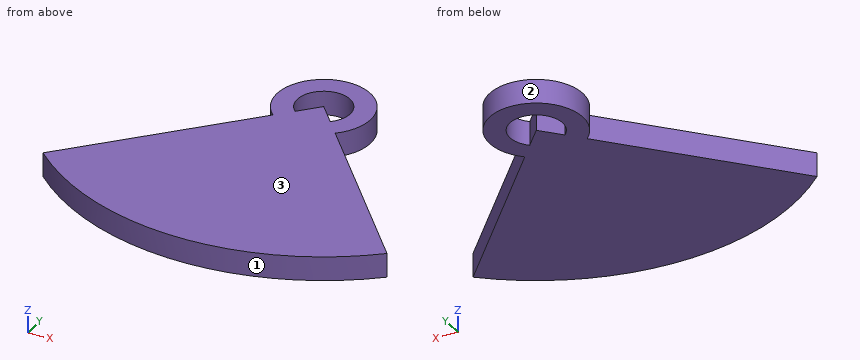
```python
from build123d import *

# Parameters (mm, degrees)
F1_DEPTH = 3
F6_DEPTH = 3


# Not quite as in the source:
# - the program builds the solid bodies; features that only make, move or delete a surface that nothing else refers to are left out


with BuildPart() as f1:
    # F0 (on Top) → F1 (new body)
    with BuildSketch(Plane.XY):
        with BuildLine():
            Line((-3.8056071322, 19.4965880074), (-21.5033702552, 0))
            ThreePointArc((-21.5033702552, 0), (0.1091537997, -8.3463338313), (21.7216778547, 0))
            Line((21.7216778547, 0), (4.0239147316, 19.4965880074))
            Line((4.0239147316, 19.4965880074), (2.3194467965, 21.374300398))
            Line((2.3194467965, 21.374300398), (0.1091537997, 23.8092506024))
            Line((0.1091537997, 23.8092506024), (-2.1011391971, 21.374300398))
            Line((-2.1011391971, 21.374300398), (-3.8056071322, 19.4965880074))
        make_face()
        with BuildLine():
            Line((-15.8273540437, 0), (0.1091537997, 23.8092506024))
            Line((0.1091537997, 23.8092506024), (16.0456616431, 0))
            ThreePointArc((16.0456616431, 0), (0.1091537997, -4.8412763821), (-15.8273540437, 0))
        make_face(mode=Mode.SUBTRACT)
        with BuildLine():
            Line((16.0456616431, 0), (0.1091537997, 23.8092506024))
            Line((0.1091537997, 23.8092506024), (-15.8273540437, 0))
            ThreePointArc((-15.8273540437, 0), (0.1091537997, -4.8412763821), (16.0456616431, 0))
        make_face()
        with BuildLine():
            Line((-10.592116043, 0), (0.1091537997, 23.8092506024))
            Line((0.1091537997, 23.8092506024), (11.3627482206, 0))
            ThreePointArc((11.3627482206, 0), (0.3853160888, -2.256488537), (-10.592116043, 0))
        make_face(mode=Mode.SUBTRACT)
        with BuildLine():
            Line((11.3627482206, 0), (0.1091537997, 23.8092506024))
            Line((0.1091537997, 23.8092506024), (-10.592116043, 0))
            ThreePointArc((-10.592116043, 0), (0.3853160888, -2.256488537), (11.3627482206, 0))
        make_face()
    extrude(amount=F1_DEPTH)

    # F0 (on Top) → F6 (join)
    with BuildSketch(Plane.XY):
        with BuildLine():
            ThreePointArc((4.0239147316, 19.4965880074), (0.1091537997, 29.6337172572), (-3.8056071322, 19.4965880074))
            Line((-3.8056071322, 19.4965880074), (-2.1011391971, 21.374300398))
            ThreePointArc((-2.1011391971, 21.374300398), (0.1091537997, 27.0977727066), (2.3194467965, 21.374300398))
            Line((2.3194467965, 21.374300398), (4.0239147316, 19.4965880074))
        make_face()
    extrude(amount=F6_DEPTH)


solid = f1.part
```
Model file for the job. Use its own axes, mm. Face numbers are marked on the shaded views. Coordinates: 2 decimals unless noted, no trailing zeros. Order: outer loops, then holes, each group sorted by start corner. A loop starts at its lowest first (then second) coordinate and runs counter-clockwise, first axis right, second up. Notation, with made-up numbers: (66.5, 0) -> (81.5, 0) arc R26 ccw to (81.5, 22) -> close; hole circle Ø6 at (39, 48.5). An arc over 180 degrees is marked (long way). Answer as a JSON object with one key per item and string values. Group by question number.
1) Cut at B-B, the plane y = 25. Write the cut outline in (x, z), then the cut area to 3 significant figures.
2) Cut at C-C, the plane x = -5. Write the cut outline in (y, z).
3) Cut at A-A, the plane z = 1.95. Write the cut outline in (x, y), then the cut area to 3 significant figures.
4) Drill centre lines: L1, parallel to Y at x = -1.5, z = 0.3; L2, parallel to Y at x = 0, z = 2.8; L3, parallel to X at y = 26, z = 0.2. Where is each one in solid material? Low to high.
5) Cut at D-D, the plane y = -3.5. Write the cut outline in (x, z).
6) Pull direction Y, two halves, no side cores. Call the marked faces 1, 2 and 3: +Y half, -Y half, draft (parallel to the pull), parting line (faces both ways), or undercut.
7) Flat gauge pin, fed straight in: pin 1 (1.5 mm diameter, centred on x = 8.5, y = 25, fed in from -Z). Where does the tip first touch, or does it go through?
Check values:
{
 "1": {"outline": "(-5.59, 0) -> (-2.96, 0) -> (-2.96, 3) -> (-5.59, 3) -> close; (3.17, 0) -> (5.81, 0) -> (5.81, 3) -> (3.17, 3) -> close", "area": "15.8 mm²"},
 "2": {"outline": "(-7.94, 0) -> (18.18, 0) -> (18.18, 3) -> (-7.94, 3) -> close; (21.01, 0) -> (26.61, 0) -> (26.61, 3) -> (21.01, 3) -> close"},
 "3": {"outline": "(-21.5, 0) arc R32.16 ccw to (21.72, 0) -> (4.02, 19.5) arc R5.82 ccw (long way) to (-3.81, 19.5) -> close; hole (-2.1, 21.37) -> (0.11, 23.81) -> (2.32, 21.37) arc R3.29 ccw (long way) to start", "area": "818 mm²"},
 "4": {"L1": "y = -8.31 to 22.04, 26.68 to 29.41", "L2": "y = -8.35 to 23.69, 27.1 to 29.63", "L3": "x = -5.29 to -2.34, 2.56 to 5.51"},
 "5": {"outline": "(-16.87, 0) -> (17.09, 0) -> (17.09, 3) -> (-16.87, 3) -> close"},
 "6": {"face 1": "-Y half", "face 2": "undercut", "face 3": "draft"},
 "7": {"pin 1": "passes through"}
}
